```python
from build123d import *

# Parameters (mm, degrees)
F3_R     = 6.985
F3_R_2   = 5.08
F4_DEPTH = 1.016


with BuildPart() as f2:
    # F1 (on Front) → F2 (revolve)
    with BuildSketch(Plane.XZ):
        with BuildLine():
            Line((252.476, 0), (0, 0))
            Line((0, 0), (0, -1.016))
            Line((0, -1.016), (252.984, -1.016))
            Line((252.984, -1.016), (252.984, -41.275))
            Line((252.984, -41.275), (254, -41.275))
            Line((254, -41.275), (254, -1.524))
            ThreePointArc((254, -1.524), (253.553631, -0.446369), (252.476, 0))
        make_face()
    revolve(axis=Axis((0, 0, -44.069175), (0, 0, -1)))

    # F3 (on Top) → F4 (cut, through all)
    with BuildSketch(Plane.XY):
        with Locations((205.490317, 66.767851)):
            Circle(F3_R)
        with Locations((0, 216.065305)):
            Circle(F3_R)
        with Locations((-205.490317, 66.767851)):
            Circle(F3_R)
        with Locations((-127, -174.800504)):
            Circle(F3_R)
        with Locations((127, -174.800504)):
            Circle(F3_R)
        Circle(F3_R_2)
    extrude(amount=-F4_DEPTH, mode=Mode.SUBTRACT)


solid = f2.part
```
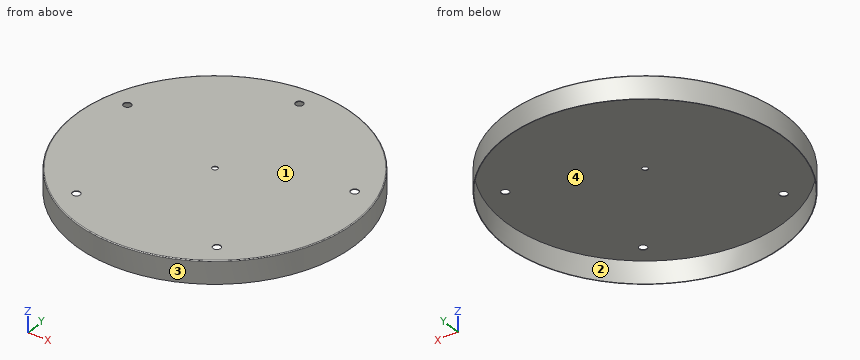
Geometry check sheet. Reference: the model listing, model coordinates, mm. Face numbers are marked on the shaded views. Coordinates: 2 decimals unless noted, no trailing zeros. Order: outer loops, then holes, each group sorted by start corner. A loop starts at its lowest first (then second) coordinate and runs counter-clockwise, first axis right, second up.
Q1. Depth check by flat-ended pin: pin 1 Ø1.5 at (y, z) = (201, -26) entering from -X; pin 2 Ø12 at (x, y) = (-148, 140) entering from -Z; pin 3 Ø10 at (x, z) = (181, -26) entering from -Y. Enter the tip coordinate at first touch or a pass-through.
Reply:
pin 1: stops at x = -156.26
pin 2: stops at z = -1.02
pin 3: stops at y = -183.14
Q2. Draft check along X on the marked faces 1, 2, 3 and 4. Enter one of: released by +X, released by -X, zero draft, split by the parting line, or undercut.
Reply:
face 1: zero draft
face 2: undercut
face 3: split by the parting line
face 4: undercut
Q3. Sectioned sample at A-A on z = -18.5. Record the cut outline in (x, y).
Reply:
outline: circle Ø508 at (0, 0); hole circle Ø505.97 at (0, 0)
Q4. Thickness scan on probe 1 along Y at (x, z) = (0, -30); probe 2 along Z at (x, y) = (-57, -113.5); probe 3 along Y at (x, z) = (117.5, -34). Record the ranges inside material, lowest first.
Reply:
probe 1: y = -254 to -252.98, 252.98 to 254
probe 2: z = -1.02 to 0
probe 3: y = -225.19 to -224.04, 224.04 to 225.19
